```python
from build123d import *

# Parameters (mm, degrees)
EXTRUDE_1_DEPTH = 1


with BuildPart() as part:
    # 草图1 → 凸台-拉伸1 (new body)
    with BuildSketch(Plane.XY):
        with BuildLine():
            Line((-61, -32), (-60.5, -32))
            ThreePointArc((-60.5, -32), (-57.671572875, -33.171572875), (-56.5, -36))
            Line((-56.5, -36), (-56.5, -36.5))
            Line((-56.5, -36.5), (-40.994977349, -36.5))
            Line((-40.994977349, -36.5), (-40.994977349, -36))
            ThreePointArc((-40.994977349, -36), (-39.823404474, -33.171572875), (-36.994977349, -32))
            Line((-36.994977349, -32), (-34.648063919, -32))
            add(Edge.make_bspline(
                [(-34.648063919, -32), (-33.649188035, -29.801521516), (-32.763169649, -27.559357), (-31.602588747, -24.130906164), (-31.243984455, -22.977553874), (-30.584883688, -20.657911853), (-30.284019718, -19.490574743), (-29.738521235, -17.141167899), (-29.493713152, -15.957957975), (-29.060766213, -13.585894928), (-28.872271639, -12.396416473), (-28.388058555, -8.817968759), (-28.173290485, -6.419025656), (-28.058899629, -4.007718216)],
                knots=[0, 0, 0, 0, 0.25, 0.25, 0.375, 0.375, 0.5, 0.5, 0.625, 0.625, 0.75, 0.75, 1, 1, 1, 1], degree=3))
            ThreePointArc((-28.058899629, -4.007718216), (-30.500861029, -2.964930185), (-31.508087081, -0.508087081))
            Line((-31.508087081, -0.508087081), (-31.508087081, -0.5))
            Line((-31.508087081, -0.5), (-77, -0.5))
            Line((-77, -0.5), (-77, -14.5))
            Line((-77, -14.5), (-61, -14.5))
            Line((-61, -14.5), (-61, -32))
        make_face()
    extrude(amount=EXTRUDE_1_DEPTH)


solid = part.part
```
Geometry check sheet. Reference: the model listing, model coordinates, mm. A direction names the side the tool comes from. Give positions to 0.01 mm unless a question says otherwise; leave off trailing zeros. Write each loop counter-clockwise with the first axis right and the second up, starting at its lowest first coordinate (ties: lowest second). Pieces come first, ordered by that corner, then holes. Notation, with made-up numbers: (-18.5, 70) - (35.5, 70) arc R7 cw to (35.5, 75) - close; hole circle Ø10 at (54.25, 58.5). An arc over 180 degrees is marked (long way). Use a Markdown table: item, result.
Q1. Set-up check for faces 1 (the face through (-47, -14, 0)), 2 (the face through (-35.8, -32, 0.5)), 3 (the face through (-61, -23.1, 0.5)): record each of +Z, -Z, +X, -X, +Y, -Y from which the full face is reachable in a straight line by a thin tool's end or side.
Computed:
| item | result |
|---|---|
| face 1 | -Z, +X, -X, +Y, -Y |
| face 2 | +Z, -Z, +X, -Y |
| face 3 | +Z, -Z, -X, -Y |
Q2. Section check A-A, the plane x = -35.5. Enter the section's corners in (y, z), then the cut area to 3 significant figures.
Computed:
| item | result |
|---|---|
| outline | (-32, 0) - (-0.5, 0) - (-0.5, 1) - (-32, 1) - close |
| area | 31.5 mm² |
Q3. Thickness scan on L1, parallel to Y at x = -68, z = 0.9; L2, parallel to Y at x = -60.5, z = 0.6; L3, parallel to X at y = -34, z = 0.9. Record the ranges inside material, lowest first. Write a range as [from, to].
Computed:
| item | result |
|---|---|
| L1 | y = [-14.5, -0.5] |
| L2 | y = [-32, -0.5] |
| L3 | x = [-57.04, -40.46] |
Q4. Section check B-B, the plane x = -67. Enter the section's corners in (y, z).
Computed:
| item | result |
|---|---|
| outline | (-14.5, 0) - (-0.5, 0) - (-0.5, 1) - (-14.5, 1) - close |
Q5. Go/stop test with flat-tipped pins: P1, Ø4, axis at x = -39, y = -22.5, coming from the -Z side; P2, Ø0.5, axis at y = -24, z = 0.5, coming from the -X side. Record where each tip stops, or that it passes through.
Computed:
| item | result |
|---|---|
| P1 | stops at z = 0 |
| P2 | stops at x = -61 |
